Autodesk Inventor part; units mm, degrees
ref_plane "YZ Plane" through (0, 0, 0) normal (1, 0, 0) x (0, 1, 0)
ref_plane "XZ Plane" through (0, 0, 0) normal (0, 1, 0) x (-1, 0, 0)
ref_plane "XY Plane" through (0, 0, 0) normal (0, 0, 1) x (1, 0, 0)
sketch "Sketch1" plane through (0, 0, 0) normal (0, 1, 0) x (-1, 0, 0)
  circle A0 centre (0, 0) radius 7.25
  line L0 (0, -7.25) -> (0, -17.25)
  circle A1 centre (0, -17.25) radius 7.25
  line L1 (0, -24.5) -> (0, -34.5)
  circle A2 centre (0, -34.5) radius 7.25
  line L2 (0, -7.25) -> (0, -10)
  line L3 (0, -24.5) -> (0, -27.25)
  line L4 (0, 7.25) -> (-16, 7.25)
  line L5 (-16, 7.25) -> (-16, 2)
  circle A3 centre (-16, 2) radius 5.25
  line L6 (0, -41.75) -> (-16, -41.75)
  line L7 (-16, -41.75) -> (-16, -36.5)
  circle A4 centre (-16, -36.5) radius 5.25
  line L8 (0, -8.625) -> (-16, -8.625)
  line L9 (0, -25.875) -> (-16, -25.875)
  circle A5 centre (-10.75, -8.625) radius 5.25
  circle A6 centre (-10.75, -25.875) radius 5.25
  line L10 (-16, 7.25) -> (-22.25, 7.25)
  line L11 (-22.25, 7.25) -> (-32.75, 7.25)
  line L12 (-32.75, 7.25) -> (-32.75, -41.75)
  line L13 (-32.75, -41.75) -> (-22.25, -41.75)
  line L14 (-22.25, -41.75) -> (-22.25, 7.25)
  line L15 (7.25, 7.25) -> (9.25, 7.25)
  line L16 (9.25, 7.25) -> (9.25, 9.25)
  line L17 (-32.75, -41.75) -> (-32.75, -43.75)
  line L18 (-32.75, -43.75) -> (-34.75, -43.75)
  line L19 (9.25, 9.25) -> (-34.75, 9.25)
  line L20 (-34.75, 9.25) -> (-34.75, -43.75)
  line L21 (-34.75, -43.75) -> (9.25, -43.75)
  line L22 (9.25, -43.75) -> (9.25, 9.25)
  dimension "d0" = 14.5
  dimension "d14" = 10
  dimension "d15" = 14.5
  dimension "d16" = 10
  dimension "d17" = 14.5
  dimension "d23" = 16
  dimension "d24" = 5.25
  dimension "d25" = 10.5
  dimension "d26" = 16
  dimension "d27" = 5.25
  dimension "d28" = 10.5
  dimension "d29" = 10.5
  dimension "d31" = 6.25
  dimension "d32" = 10.5
  dimension "d33" = 2
  dimension "d34" = 2
  dimension "d35" = 2
  dimension "d36" = 2
extrude "Extrusion1" add sketch "Sketch1" along normal blind 12
sketch "Sketch2" plane through (0, 0, 0) normal (0, -1, 0) x (1, 0, 0)
  line L0 (34.75, 9.25) -> (34.75, -43.75)
  line L1 (34.75, 9.25) -> (-9.25, 9.25)
  line L2 (-9.25, 9.25) -> (-9.25, -43.75)
  line L3 (-9.25, -43.75) -> (34.75, -43.75)
  line L4 (34.75, -43.75) -> (34.75, 9.25)
  point P0 (0, 0)
extrude "Extrusion2" add sketch "Sketch2" along normal blind 3
sketch "Sketch3" plane through (0, 12, 0) normal (0, 1, 0) x (1, 0, 0)
  line L0 (32.75, 41.75) -> (32.75, -7.25)
  line L1 (32.75, 41.75) -> (34.75, 41.75)
  line L2 (34.75, -9.25) -> (34.75, 43.75)
  line L3 (32.75, -7.25) -> (34.75, -7.25)
  line L4 (34.75, -7.25) -> (34.75, 41.75)
  line L5 (34.75, 41.75) -> (32.75, 41.75)
  line L6 (32.75, 41.75) -> (32.75, -7.25)
  point P0 (0, 0)
extrude "Extrusion3" cut sketch "Sketch3" against normal blind 7
fillet "Fillet1" radius 7 1 edges at (34.75, 12, 8.25)
fillet "Fillet2" radius 7 1 edges at (34.75, 12, -42.75)
sketch "Sketch4" plane through (0, 12, 0) normal (0, 1, 0) x (1, 0, 0)
  line L0 (22.25, 41.75) -> (27.75, 41.75)
  line L1 (22.25, 41.75) -> (22.25, 31.25)
  line L2 (22.25, -7.25) -> (22.25, 41.75)
  line L3 (22.25, -7.25) -> (22.25, 3.25)
  line L4 (16, 17.25) -> (22.25, 31.25)
  line L5 (16, 17.25) -> (22.25, 3.25)
  line L6 (22.25, 17.25) -> (13.25, 17.25)
  line L7 (13.25, 17.25) -> (22.25, 31.25)
  line L8 (13.25, 17.25) -> (22.25, 3.25)
  line L9 (22.25, 31.25) -> (22.25, 3.25)
  point P0 (0, 0)
  dimension "d45" = 10.5
  dimension "d46" = 9
extrude "Extrusion4" cut sketch "Sketch4" against normal blind 12 contours L6 L4 L2
extrude "Extrusion5" cut sketch "Sketch4" against normal blind 12 contours L5 L6 L2
extrude "Extrusion6" cut sketch "Sketch4" against normal blind 12 contours L8 L6 L5
extrude "Extrusion7" cut sketch "Sketch4" against normal through all contours L6 L7 L4
sketch "Sketch5" plane through (0, -3, 0) normal (0, -1, 0) x (1, 0, 0)
  line L0 (34.75, 9.25) -> (-9.25, 9.25)
  line L1 (-9.25, 9.25) -> (-9.25, -43.75)
  line L2 (-9.25, -43.75) -> (34.75, -43.75)
  line L3 (34.75, -43.75) -> (34.75, 9.25)
  point P0 (0, 0)
extrude "Extrusion8" add sketch "Sketch5" against normal blind 3
fillet "Fillet3" radius 10 1 edges at (22.25, 6, -31.25)
fillet "Fillet4" radius 10 1 edges at (22.25, 6, -3.25)
fillet "Fillet5" radius 10 1 edges at (13.25, 6, -17.25)
sketch "Sketch6" plane through (-9.25, -3, 9.25) normal (0, 0, 1) x (1, 0, 0)
  point P0 (9.25, 3)
sketch "Sketch7" plane through (0, 12, 0) normal (0, 1, 0) x (1, 0, 0)
  point P0 (0, 0)
fillet "Fillet6" radius 8 1 edges at (-9.25, 4.5, 9.25)
fillet "Fillet7" radius 8 1 edges at (-9.25, 4.5, -43.75)
fillet "Fillet8" radius 1 7 edges at (32.6997, 9.9497, 9.25) (13.25, 12, 9.25) (-6.9069, 12, 6.9069) (-6.9069, 12, -41.4069) (32.6997, 9.9497, -43.75) (34.75, 1, -43.75) (34.75, 1, 9.25)
properties part number "multi_battery_holder_3DPrint"
The listing builds one solid part. Answer for the finished solid, in the listing's coordinates (mm). Round coordinates to 2 decimals unless told otherwise and drop trailing zeros. Loops run counter-clockwise (first coordinate to the right, second up) from the corner with the lowest first, then second, coordinate; pieces in that order, holes last. Notation, with made-up numbers: (-8, 78) - (51, 78) arc R32 ccw to (51, 111) - close; hole circle Ø2 at (59, 89.5). An arc over 180 degrees is marked (long way). Use one line per item in the form item = value. Start each with the question number.
1. Consider line 1 (Z direction, x = 0, y = 6.5); line 2 (Z direction, x = 10.5, y = 6.5); line 3 (X direction, y = 3.75, z = -9.5). Determine where each line is inside the solid, lowest interval first. Write a range as [from, to].
2. The part is cut by section B-B on y = 1.5. Give the number of separate pieces and of enclosed holes in the cut face, then the cut area to 3 significant figures.
3. Given pin 1 Ø2 at (x, z) = (-4.5, -38) entering from +Y, flat-ended and moving along its own axis, determine where the tip first touches the part or whether it passes through.
4. The part is cut by section A-A on x = 26. Determine the outline of the cut face in (y, z).
5. The part is cut by section C-C on z = -17.25. Determine the outline of the cut face in (x, y).
6. The part is cut by section D-D on z = -32. Determine the outline of the cut face in (x, y).
7. For a pull along Z with two mould halves and no side action, classify faces 1 (the face through (0, 0, -17)), 2 (the face through (-9.25, 4, -18)), 3 (the face through (1.57, 5.92, -27.42)) as pulls with the +Z half, pulls with the -Z half, needs draft (parallel to the pull), parting line crosses it, or undercut.
Geometry check:
q1.line_1 = [-43.75, -41.75], [-27.25, -24.5], [-10, -7.25], [7.25, 9.25]
q1.line_2 = [-43.75, -31.12], [-20.63, -13.87], [-3.38, 9.25]
q1.line_3 = [-9.25, 5.57], [15.93, 18.23], [32.75, 34.75]
q2.separate_pieces = 1
q2.enclosed_holes = 8
q2.area = 827 mm^2
q3.pin_1 = 0
q4.outline = (-3, -43.75) - (11, -43.75) arc R1 ccw to (12, -42.75) - (12, -41.75) - (0, -41.75) - (0, 7.25) - (12, 7.25) - (12, 8.25) arc R1 ccw to (11, 9.25) - (-3, 9.25) - close
q5.outline = (-9.25, -3) - (34.75, -3) - (34.75, 5) - (32.75, 5) - (32.75, 0) - (15.14, 0) - (15.14, 12) - (7.25, 12) - (7.25, 0) - (-7.25, 0) - (-7.25, 12) - (-8.25, 12) arc R1 ccw to (-9.25, 11) - close
q6.outline = (-9.25, -3) - (34.75, -3) - (34.75, 5) - (32.75, 5) - (32.75, 0) - (22.01, 0) - (22.01, 12) - (18.7, 12) - (18.7, 0) - (13.3, 0) - (13.3, 12) - (6.81, 12) - (6.81, 0) - (-6.81, 0) - (-6.81, 12) - (-8.25, 12) arc R1 ccw to (-9.25, 11) - close
q7.face_1 = undercut
q7.face_2 = needs draft
q7.face_3 = undercut
